from build123d import *

# Parameters (mm, degrees)
SKETCH1_W               = 18.796
SKETCH1_H               = 11.303
BASE_DEPTH              = 6.35
BOXSLOTS_DEPTH          = 2.286
MOUTINGHOLE_D           = 3.6576
MOUTINGHOLE_CBORE_D     = 7.14502
MOUTINGHOLE_CBORE_DEPTH = 3.5052


with BuildPart() as part:
    # Sketch1 → Base (new body)
    with BuildSketch(Plane(origin=(0, 0, 0), x_dir=(1, 0, 0), z_dir=(0, 1, 0))):
        Rectangle(SKETCH1_W, SKETCH1_H)
    extrude(amount=BASE_DEPTH)

    # Sketch2 → BoxSlots (cut)
    with BuildSketch(Plane.XZ):
        with BuildLine():
            Line((-4.937125, 5.6515), (-4.937125, 4.1783))
            ThreePointArc((-4.937125, 4.1783), (-5.334, 3.781425), (-5.730875, 4.1783))
            Line((-5.730875, 4.1783), (-5.730875, 5.6515))
            ThreePointArc((-5.730875, 5.6515), (-5.334, 6.048375), (-4.937125, 5.6515))
        make_face()
        with BuildLine():
            Line((5.730875, 5.6515), (5.730875, 4.1783))
            ThreePointArc((5.730875, 4.1783), (5.334, 3.781425), (4.937125, 4.1783))
            Line((4.937125, 4.1783), (4.937125, 5.6515))
            ThreePointArc((4.937125, 5.6515), (5.334, 6.048375), (5.730875, 5.6515))
        make_face()
    extrude(amount=-BOXSLOTS_DEPTH, mode=Mode.SUBTRACT)

    # MoutingHole (through all)
    with Locations(Plane(origin=(0, 6.35, 0), x_dir=(1, 0, 0), z_dir=(0, 1, 0))):
        with Locations((0, 0)):
            CounterBoreHole(MOUTINGHOLE_D / 2, MOUTINGHOLE_CBORE_D / 2, MOUTINGHOLE_CBORE_DEPTH)


solid = part.part
The listing builds one solid part. Answer for the finished solid, in the listing's coordinates (mm). A direction names the side the tool comes from. Round coordinates to 2 decimals unless told otherwise and drop trailing zeros. Loops run counter-clockwise (first coordinate to the right, second up) from the corner with the lowest first, then second, coordinate; pieces in that order, holes last. Notation, with made-up numbers: M -2,88.25 L 37,88.25 A18 cw 37,97.25 Z; hole C 14,72 d3. An arc over 180 degrees is marked long. Write each question's results on one line, items separated by ' | '. Start each with the question number.
1) Which of the six approach directions +Z, -Z, +X, -X, +Y, -Y give full straight-line access (tool end or side, diameter ignored) to faces 1 (the flat face through (0, 3, -5.652)), 2 (the flat face through (5.731, 1, 5)), 3 (the cylindrical face through (-2.633, 4.622, -2.414))?
2) Find section A-A on z = 0. Write down the section's boundary in (x, y).
3) Find section B-B on x = 0. Write down the section's boundary in (y, z), plus the area to 3 significant figures.
4) Determine the mould class of faces 4 (the flat face through (-2, 0, 0)), 5 (the flat face through (-9.398, 3, 0)), 6 (the flat face through (-2, 2.845, -1)) for opening direction X: pulls with the +X half, pulls with the -X half, needs draft (parallel to the pull), parting line crosses it, or undercut.
5) Find section C-C on y = 4.5. Write down the section's boundary in (x, z).
6) Straight lines are drawn through the part: probe 1 along X at (y, z) = (0.5, 4.25); probe 2 along Z at (x, y) = (0, 5.3); probe 3 along Z at (x, y) = (0, 0.9). For each, find the intervals that lie inside material, in ascending order.
7) Find section D-D on z = 5. Write down the section's boundary in (x, y).
8) Each of these flat-tipped pins is pushed along its axis until it touches: pin 1 (3.5 mm diameter, centred on x = 0, z = 0, fed in from +Y); pin 2 (5.5 mm diameter, centred on x = 0, z = 0, fed in from +Y). Where does it stop, or does it pass through?
Final values:
1) face 1: -Z, +X, -X, +Y, -Y | face 2: +Z, -Y | face 3: +Y
2) outline: M -9.4,0 L -1.83,0 L -1.83,2.84 L -3.57,2.84 L -3.57,6.35 L -9.4,6.35 Z; M 1.83,0 L 9.4,0 L 9.4,6.35 L 3.57,6.35 L 3.57,2.84 L 1.83,2.84 Z
3) outline: M 0,-5.65 L 6.35,-5.65 L 6.35,-3.57 L 2.84,-3.57 L 2.84,-1.83 L 0,-1.83 Z; M 0,1.83 L 2.84,1.83 L 2.84,3.57 L 6.35,3.57 L 6.35,5.65 L 0,5.65 Z | area: 36.3 mm²
4) face 4: needs draft | face 5: pulls with the -X half | face 6: undercut
5) outline: M -9.4,-5.65 L 9.4,-5.65 L 9.4,5.65 L -9.4,5.65 Z; hole C 0,0 d7.15
6) probe 1: -9.4 to -5.73, -4.94 to 4.94, 5.73 to 9.4 | probe 2: -5.65 to -3.57, 3.57 to 5.65 | probe 3: -5.65 to -1.83, 1.83 to 5.65
7) outline: M -9.4,0 L -5.73,0 L -5.73,2.29 L -4.94,2.29 L -4.94,0 L 4.94,0 L 4.94,2.29 L 5.73,2.29 L 5.73,0 L 9.4,0 L 9.4,6.35 L -9.4,6.35 Z
8) pin 1: through | pin 2: y = 2.84
